Input: part model. Units: mm. Frame: model coordinates. Face numbers are marked on the shaded views. A direction names the side the tool comes from. Round coordinates to 2 decimals unless told otherwise and drop trailing zeros. Order: outer loops, then holes, each group sorted by start corner. A loop starts at its lowest first (then second) coordinate and runs counter-clockwise, first axis right, second up.
Item 1: Reachability of the marked faces 1, 2, 3, 4 and 5 from +Z, -Z, +X, -X, +Y, -Y: full face, straight path, thin tool, end or side. Return the list, or none.
Item 2: Mould query, pull axis X, two halves, no side actions, for the marked faces 6, 7 and 8. Classes: released by +X, released by -X, zero draft, split by the parting line, or undercut.
Item 3: Cut plane D-D on z = -27. Output: boundary loops of the cut face in (x, y), then the cut area to 3 significant figures.
Item 4: Cut plane B-B on z = -10.5. Give the number of separate pieces and of enclosed holes in the cut face, then the cut area to 3 significant figures.
Item 5: First-contact query: pin 1 (3 mm diameter, centred on y = 31.5, z = -22.5, fed in from -X); pin 2 (12 mm diameter, centred on x = 0.5, y = 7, fed in from +Z); pin 3 (8 mm diameter, centred on y = 16, z = -2.5, fed in from +X); pin 4 (2.5 mm diameter, centred on x = -14.22, z = -19.03, fed in from -Y). Flat tips, straight axial feed; report the tip coordinate or a pass-through.
Item 6: Cut plane C-C on y = 6.5. Output: boundary loops of the cut face in (x, z).
Item 7: Cut plane A-A on x = -6. Output: boundary loops of the cut face in (y, z).
Item 8: Line query: L1, parallel to X at y = 33.5, z = -23.5; L2, parallel to Y at x = 0, z = -14.5; L3, parallel to Y at x = -14, z = -13. Output: solid intervals per line, ascending.
```python
from build123d import *

# Parameters (mm, degrees)
BOSS_EXTRUDE1_DEPTH = 24
BOSS_EXTRUDE2_DEPTH = 8
SKETCH2_R           = 2
BOSS_EXTRUDE3_DEPTH = 2
SKETCH3_R           = 2
CUT_EXTRUDE1_DEPTH  = 37.612003683
BOSS_EXTRUDE4_DEPTH = 24
SKETCH6_R           = 2
BOSS_EXTRUDE5_DEPTH = 4
CUT_EXTRUDE2_DEPTH  = 4
CUT_EXTRUDE4_DEPTH  = 59.761051842


with BuildPart() as part:
    # Sketch1 → Boss-Extrude1 (new body)
    with BuildSketch(Plane.XY):
        Polygon((-18.223289316, 0), (-16.691476591, 0), (25.776710684, 0), (25.776710684, 2), (19.776710684, 2), (16.776710684, 2), (-7.223289316, 2), (-10.223289316, 2), (-18.223289316, 2), align=None)
    extrude(amount=-BOSS_EXTRUDE1_DEPTH)

    # Sketch1_4 → Boss-Extrude2 (add)
    with BuildSketch(Plane.XY):
        with BuildLine():
            Line((16.776710684, 2), (19.776710684, 2))
            ThreePointArc((19.776710684, 2), (17.655390341, 2.878679656), (16.776710684, 5))
            Line((16.776710684, 5), (16.776710684, 12))
            Line((16.776710684, 12), (-7.223289316, 12))
            Line((-7.223289316, 12), (-7.223289316, 5))
            ThreePointArc((-7.223289316, 5), (-8.101968972, 2.878679656), (-10.223289316, 2))
            Line((-10.223289316, 2), (-7.223289316, 2))
            Line((-7.223289316, 2), (16.776710684, 2))
        make_face()
    extrude(amount=-BOSS_EXTRUDE2_DEPTH)

    # Sketch2 → Boss-Extrude3 (add)
    with BuildSketch(Plane(origin=(0, 2, 0), x_dir=(1, 0, 0), z_dir=(0, 1, 0))):
        with BuildLine():
            Line((-18.223289316, 0), (-10.223289316, 0))
            Line((-10.223289316, 0), (-10.223289316, -8))
            ThreePointArc((-10.223289316, -8), (-14.223289316, -12), (-18.223289316, -8))
            Line((-18.223289316, -8), (-18.223289316, 0))
        make_face()
        with Locations(Location((-14.223289316, -8, 0), (0, 0, 180))):
            Circle(SKETCH2_R, mode=Mode.SUBTRACT)
    extrude(amount=-BOSS_EXTRUDE3_DEPTH)

    # Sketch3 → Cut-Extrude1 (cut, through all)
    with BuildSketch(Plane(origin=(0, 2, 0), x_dir=(1, 0, 0), z_dir=(0, 1, 0))):
        with Locations(Location((21.776710684, 3.027714233, 0), (0, 0, 180))):
            Circle(SKETCH3_R)
        with Locations(Location((21.776710684, 19.027714233, 0), (0, 0, 180))):
            Circle(SKETCH3_R)
        with Locations(Location((-14.223289316, 19.027714233, 0), (0, 0, 180))):
            Circle(SKETCH3_R)
    extrude(amount=-CUT_EXTRUDE1_DEPTH, mode=Mode.SUBTRACT)

    # Sketch5 → Boss-Extrude4 (add)
    with BuildSketch(Plane(origin=(16.776710684, 0, 0), x_dir=(0, 0, -1), z_dir=(1, 0, 0))):
        Polygon((8, 12), (0, 12), (22.505945882, 36.134672153), (38.505945882, 36.134672153), (38.505945882, 32.134672153), (24.245195382, 32.134672153), (19.201196493, 26.725645572), (8, 14.713832938), align=None)
    extrude(amount=-BOSS_EXTRUDE4_DEPTH)

    # Sketch6 → Boss-Extrude5 (add)
    # profile 1 of 2: a face of its own
    with BuildSketch(Plane(origin=(0, 5.581461158, 5.985384302), x_dir=(1, 0, 0), z_dir=(0, 0.6819983600624966, 0.7313537016191722))):
        with BuildLine():
            Line((-7.223289316, 18.776244419), (-11.223289316, 18.776244419))
            ThreePointArc((-11.223289316, 18.776244419), (-17.223289316, 24.776244419), (-11.223289316, 30.776244419))
            Line((-11.223289316, 30.776244419), (-7.223289316, 30.776244419))
            Line((-7.223289316, 30.776244419), (-7.223289316, 18.776244419))
        make_face()
        with Locations(Location((-11.223289316, 24.776244419, 0), (0, 0, 270))):
            Circle(SKETCH6_R, mode=Mode.SUBTRACT)
    # profile 2 of 2: a face of its own
    with BuildSketch(Plane(origin=(0, 5.581461158, 5.985384302), x_dir=(1, 0, 0), z_dir=(0, 0.6819983600624966, 0.7313537016191722))):
        with BuildLine():
            Line((10.776710684, 32.776244419), (10.776710684, 18.776244419))
            ThreePointArc((10.776710684, 18.776244419), (8.776710684, 16.776244419), (6.776710684, 18.776244419))
            Line((6.776710684, 18.776244419), (6.776710684, 32.776244419))
            ThreePointArc((6.776710684, 32.776244419), (8.776710684, 34.776244419), (10.776710684, 32.776244419))
        make_face()
    extrude(amount=-BOSS_EXTRUDE5_DEPTH)

    # Sketch6_5 → Cut-Extrude2 (cut)
    with BuildSketch(Plane(origin=(0, 5.581461158, 5.985384302), x_dir=(1, 0, 0), z_dir=(0, 0.6819983600624966, 0.7313537016191722))):
        with BuildLine():
            Line((10.776710684, 32.776244419), (10.776710684, 18.776244419))
            ThreePointArc((10.776710684, 18.776244419), (8.776710684, 16.776244419), (6.776710684, 18.776244419))
            Line((6.776710684, 18.776244419), (6.776710684, 32.776244419))
            ThreePointArc((6.776710684, 32.776244419), (8.776710684, 34.776244419), (10.776710684, 32.776244419))
        make_face()
    extrude(amount=-CUT_EXTRUDE2_DEPTH, mode=Mode.SUBTRACT)

    # Sketch7 → Cut-Extrude4 (cut, through all)
    with BuildSketch(Plane(origin=(0, 36.134672153, 0), x_dir=(1, 0, 0), z_dir=(0, 1, 0))):
        with BuildLine():
            Line((-1.223289316, 38.505945882), (10.776710684, 38.505945882))
            ThreePointArc((10.776710684, 38.505945882), (4.776710684, 32.505945882), (-1.223289316, 38.505945882))
        make_face()
    extrude(amount=-CUT_EXTRUDE4_DEPTH, mode=Mode.SUBTRACT)


solid = part.part
```
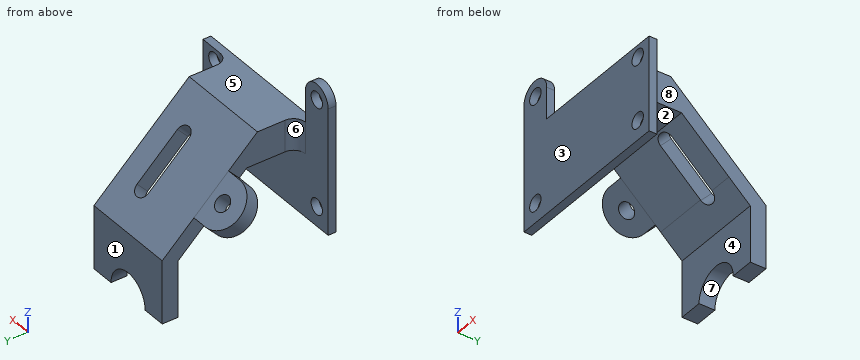
From the geometry:
1. face 1: +Z, -Z, +X, -X, +Y
1. face 2: -Z, +X, -X
1. face 3: +Z, -Z, +X, -X, -Y
1. face 4: -Z, +X, -X, -Y
1. face 5: +Z, +X, +Y, -Y
2. face 6: released by -X
2. face 7: undercut
2. face 8: released by +X
3. outline: (-7.22, 32.13) - (16.78, 32.13) - (16.78, 36.13) - (-7.22, 36.13) - close
3. area: 96.0 mm2
4. separate pieces: 3
4. enclosed holes: 0
4. area: 254 mm2
5. pin 1: stops at x = -7.22
5. pin 2: stops at z = 0
5. pin 3: stops at x = 16.78
5. pin 4: passes through
6. outline: (-7.22, -8) - (16.78, -8) - (16.78, 0) - (-7.22, 0) - close
7. outline: (0, -24) - (2, -24) - (2, -8) - (14.71, -8) - (32.13, -24.25) - (32.13, -38.51) - (36.13, -38.51) - (36.13, -22.51) - (12, 0) - (0, 0) - close
8. L1: x = -7.22 to 16.78
8. L2: y = 0 to 2, 21.68 to 27.55
8. L3: y = 0 to 2, 20.08 to 25.94
